```python
from build123d import *
from build123d import SkipClean  # not in build123d's __all__

# Parameters (mm, degrees)
F1_DEPTH      = 8
F3_DEPTH      = 8.2965155193
F3_DEPTH_BACK = 8.2965155193
F4_R          = 2.5
F5_DEPTH      = 12.5


with BuildPart() as f1:
    # F0 (on Front) → F1 (new body)
    with BuildSketch(Plane.XZ):
        with BuildLine():
            Line((20.0802286013, 8.2965155193), (-20.0802286013, 8.2965155193))
            ThreePointArc((-20.0802286013, 8.2965155193), (-25.7931508501, 5.7833391211), (-28.1397494181, 0))
            Line((-28.1397494181, 0), (-22.0952286013, 0))
            ThreePointArc((-22.0952286013, 0), (-20.0802286013, 2.015), (-18.0652286013, 0))
            Line((-18.0652286013, 0), (18.0652286013, 0))
            ThreePointArc((18.0652286013, 0), (20.0802286013, 2.015), (22.0952286013, 0))
            Line((22.0952286013, 0), (28.3767441206, 0))
            ThreePointArc((28.3767441206, 0), (25.9467509852, 5.8665223839), (20.0802286013, 8.2965155193))
        make_face()
        with BuildLine():
            Line((-22.0952286013, 0), (-28.1397494181, 0))
            ThreePointArc((-28.1397494181, 0), (-25.7931508501, -5.7833391211), (-20.0802286013, -8.2965155193))
            Line((-20.0802286013, -8.2965155193), (20.0802286013, -8.2965155193))
            ThreePointArc((20.0802286013, -8.2965155193), (25.9467509852, -5.8665223839), (28.3767441206, 0))
            Line((28.3767441206, 0), (22.0952286013, 0))
            ThreePointArc((22.0952286013, 0), (20.0802286013, -2.015), (18.0652286013, 0))
            Line((18.0652286013, 0), (-18.0652286013, 0))
            ThreePointArc((-18.0652286013, 0), (-20.0802286013, -2.015), (-22.0952286013, 0))
        make_face()
    extrude(amount=F1_DEPTH)

    # F2 (on Top) → F3 (join, two sides)
    with BuildSketch(Plane.XY) as f3_sk:
        with BuildLine():
            Line((2.4494897428, 0), (13.0258305651, 0))
            ThreePointArc((13.0258305651, 0), (0, 5.5), (-13.0258305651, 0))
            Line((-13.0258305651, 0), (-2.4494897428, 0))
            ThreePointArc((-2.4494897428, 0), (-0.251272405, 2.9873403825), (2.5, 0.5))
            ThreePointArc((2.5, 0.5), (2.4873403825, 0.248727595), (2.4494897428, 0))
        make_face()
    extrude(amount=F3_DEPTH)
    extrude(f3_sk.sketch, amount=-F3_DEPTH_BACK)

    # F4 (on Top) → F5 (cut, symmetric)
    with BuildSketch(Plane.XY):
        with Locations((0, 0.5)):
            Circle(F4_R)
    with SkipClean():  # cleaning this boolean's faces spoils the solid; the shape is the same uncleaned
        extrude(amount=F5_DEPTH, both=True, mode=Mode.SUBTRACT)


solid = f1.part
```
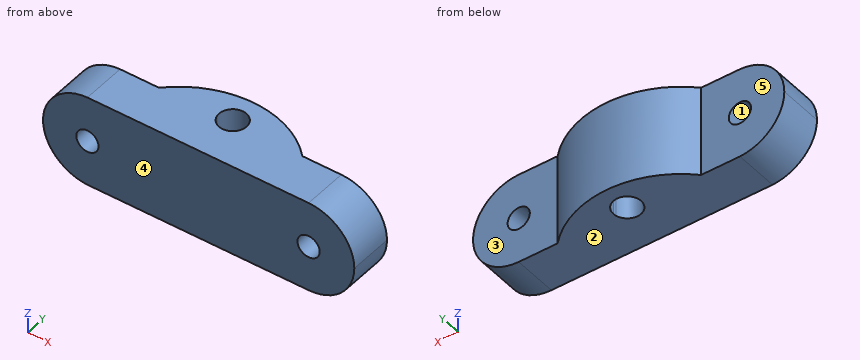
Geometry check sheet. Reference: the model listing, model coordinates, mm. Face numbers are marked on the shaded views. A direction names the side the tool comes from. Coordinates: 2 decimals unless noted, no trailing zeros. Loops run counter-clockwise (first coordinate to the right, second up) from the corner with the lowest first, then second, coordinate; pieces in that order, holes last. Notation, with made-up numbers: (-25, -13.5) -> (19, -13.5) arc R34 cw to (19, 19.5) -> close; hole circle Ø8 at (-15, -27.75). An arc over 180 degrees is marked (long way). Put each result on its own line as item: value.
1) Release check for a two-part mould opening along Z. For the marked faces 1, 2 and 3 record: released by +Z, released by -Z, zero draft, split by the parting line, or undercut.
Result set:
face 1: undercut
face 2: released by -Z
face 3: zero draft
2) Gauge pin test, flat ends, axial feed: pin 1 Ø4 at (x, z) = (-21, 4) entering from +Y; pin 2 Ø3 at (y, z) = (-3, 2.5) entering from +X; pin 3 Ø1 at (y, z) = (-5.5, -5.5) entering from +X. Record the tip position at first contact, or that the pin passes through.
Result set:
pin 1: stops at y = 0
pin 2: stops at x = 28.32
pin 3: stops at x = 26.7
3) Cross-section at D-D on x = -19.5. Record the boundary of the cut face in (y, z), plus the area to 3 significant figures.
Result set:
outline: (-8, -8.3) -> (0, -8.3) -> (0, -1.93) -> (-8, -1.93) -> close; (-8, 1.93) -> (0, 1.93) -> (0, 8.3) -> (-8, 8.3) -> close
area: 102 mm^2
4) Thickness scan on line 1 (X direction, y = -2.5, z = 1); line 2 (X direction, y = 2.5, z = 2.5); line 3 (X direction, y = -2.75, z = -1.5). Record the ranges inside material, lowest first.
Result set:
line 1: x = -28.08 to -21.83, -18.33 to 18.33, 21.83 to 28.32
line 2: x = -10 to -1.5, 1.5 to 10
line 3: x = -28 to -21.43, -18.73 to 18.73, 21.43 to 28.24
5) Cross-section at B-B on z = 0.75. Record the boundary of the cut face in (x, y), plus the area to 3 significant figures.
Result set:
outline: (-28.11, -8) -> (-21.95, -8) -> (-21.95, 0) -> (-28.11, 0) -> close; (-18.21, -8) -> (18.21, -8) -> (18.21, 0) -> (13.03, 0) arc R18.17 ccw to (-13.03, 0) -> (-18.21, 0) -> close; (21.95, -8) -> (28.34, -8) -> (28.34, 0) -> (21.95, 0) -> close; hole circle Ø5 at (0, 0.5)
area: 471 mm^2
6) Cross-section at C-C on z = -5.75. Record the boundary of the cut face in (x, y), plus the area to 3 significant figures.
Result set:
outline: (-25.83, -8) -> (26.06, -8) -> (26.06, 0) -> (13.03, 0) arc R18.17 ccw to (-13.03, 0) -> (-25.83, 0) -> close; hole circle Ø5 at (0, 0.5)
area: 494 mm^2
7) Tool access check on the marked faces 4 and 5. Record the directions out of +Z, -Z, +X, -X, +Y, -Y that give a thin tool (end or side, any length) a straight path to the whole face; none if there is none.
Result set:
face 4: +Z, -Z, +X, -X, -Y
face 5: +Z, -Z, -X, +Y
8) Cross-section at A-A on x = 0. Record the boundary of the cut face in (y, z), plus the area to 3 significant figures.
Result set:
outline: (-8, -8.3) -> (-2, -8.3) -> (-2, 8.3) -> (-8, 8.3) -> close; (3, -8.3) -> (5.5, -8.3) -> (5.5, 8.3) -> (3, 8.3) -> close
area: 141 mm^2
